Part model, mm, in its own coordinate system. Face numbers are marked on the shaded views. A direction names the side the tool comes from. Round coordinates to 2 decimals unless told otherwise and drop trailing zeros. Loops run counter-clockwise (first coordinate to the right, second up) from the corner with the lowest first, then second, coordinate; pieces in that order, holes last. Notation, with made-up numbers: (74, 50) - (99, 50) arc R28 cw to (99, 75) - close; hole circle Ø9 at (20, 45). An arc over 180 degrees is marked (long way). Put each result on its own line as item: value.
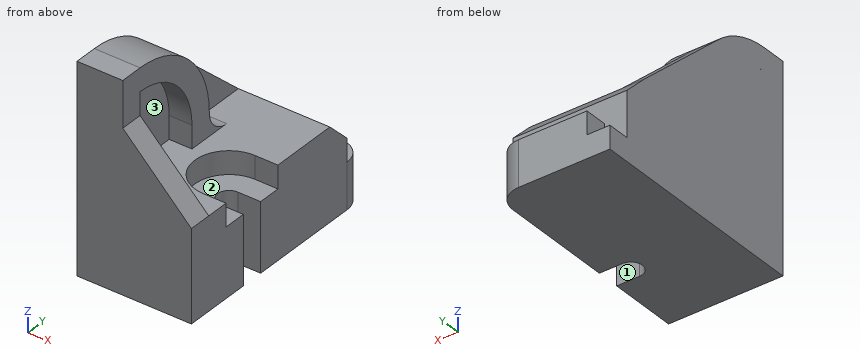
from build123d import *

# Parameters (mm, degrees)
BOSS_EXTRUDE1_DEPTH = 4
CUT_EXTRUDE1_DEPTH  = 1
SKETCH3_W           = 1
SKETCH3_H           = 1
CUT_EXTRUDE2_DEPTH  = 3
SKETCH4_W           = 2
SKETCH4_H           = 1
CUT_EXTRUDE4_DEPTH  = 6
CUT_EXTRUDE5_DEPTH  = 6
BOSS_EXTRUDE2_DEPTH = 1
BOSS_EXTRUDE3_DEPTH = 2
BOSS_EXTRUDE4_DEPTH = 1


with BuildPart() as part:
    # Sketch1 → Boss-Extrude1 (new body)
    with BuildSketch(Plane.XY):
        with BuildLine():
            Line((0, 9), (5, 9))
            ThreePointArc((5, 9), (4.707106781, 9.707106781), (4, 10))
            Line((4, 10), (0, 10))
            Line((0, 10), (0, 9))
        make_face()
        with BuildLine():
            ThreePointArc((4, 4), (3.5, 3.5), (4, 3))
            Line((4, 3), (5, 3))
            Line((5, 3), (5, 0))
            Line((5, 0), (0, 0))
            Line((0, 0), (0, 9))
            Line((0, 9), (5, 9))
            Line((5, 9), (5, 4))
            Line((5, 4), (4, 4))
        make_face()
    extrude(amount=BOSS_EXTRUDE1_DEPTH)

    # Sketch2 → Cut-Extrude1 (cut)
    with BuildSketch(Plane.XY.offset(4)):
        with BuildLine():
            Line((5, 3), (5, 2))
            Line((5, 2), (4, 2))
            ThreePointArc((4, 2), (2.5, 3.5), (4, 5))
            Line((4, 5), (5, 5))
            Line((5, 5), (5, 4))
            Line((5, 4), (4, 4))
            ThreePointArc((4, 4), (3.5, 3.5), (4, 3))
            Line((4, 3), (5, 3))
        make_face()
    extrude(amount=-CUT_EXTRUDE1_DEPTH, mode=Mode.SUBTRACT)

    # Sketch3 → Cut-Extrude2 (cut)
    with BuildSketch(Plane.XY.offset(4)):
        with Locations((0.5, 9.5)):
            Rectangle(SKETCH3_W, SKETCH3_H)
    extrude(amount=-CUT_EXTRUDE2_DEPTH, mode=Mode.SUBTRACT)

    # Sketch4 → Cut-Extrude4 (cut, through all)
    with BuildSketch(Plane.ZY):
        with Locations((3, 9.5)):
            Rectangle(SKETCH4_W, SKETCH4_H)
    extrude(amount=-CUT_EXTRUDE4_DEPTH, mode=Mode.SUBTRACT)

    # Sketch5 → Cut-Extrude5 (cut, through all)
    with BuildSketch(Plane(origin=(5, 0, 0), x_dir=(0, 0, -1), z_dir=(1, 0, 0))):
        Polygon((-3, 9), (-4, 8), (-4, 9), align=None)
    extrude(amount=-CUT_EXTRUDE5_DEPTH, mode=Mode.SUBTRACT)

    # Sketch6 → Boss-Extrude2 (add)
    with BuildSketch(Plane.XZ):
        Polygon((0, 4), (0, 9), (2, 9), (2, 7), (5, 4), align=None)
    extrude(amount=-BOSS_EXTRUDE2_DEPTH)

    # Sketch7 → Boss-Extrude3 (add)
    with BuildSketch(Plane.ZY):
        with BuildLine():
            Line((8, 1), (9, 1))
            ThreePointArc((9, 1), (7.828427125, 3.828427125), (5, 5))
            ThreePointArc((5, 5), (4.292893219, 5.292893219), (4, 6))
            Line((4, 6), (4, 4))
            Line((4, 4), (5, 4))
            ThreePointArc((5, 4), (7.121320344, 3.121320344), (8, 1))
        make_face()
    extrude(amount=-BOSS_EXTRUDE3_DEPTH)

    # Sketch9 → Boss-Extrude4 (add)
    with BuildSketch(Plane.ZY):
        Polygon((4, 8), (7.828427125, 3.828427125), (8, 1), (4, 1), align=None)
    extrude(amount=-BOSS_EXTRUDE4_DEPTH)


solid = part.part
1. Probe line 1 along Z through (x, y) = (4.05, 7); line 2 along Z through (x, y) = (1.9, 3.25); line 3 along X through (y, z) = (3.75, 4.75). List the from-to ranges inside material, lowest first. Write a range as [from, to].
A:
line 1: z = [0, 4]
line 2: z = [0, 4], [6.98, 8.31]
line 3: x = [0, 1]
2. Pin check, flat tips, straight feed: P1, Ø0.8, axis at x = 4.5, z = 3.5, coming from the +Y side; P2, Ø0.5, axis at y = 9.5, z = 1.5, coming from the -X side; P3, Ø0.8, axis at x = 4.5, z = 2, coming from the +Y side (3 decimals). Stop position of each tip, or through.
A:
P1: stops at y = 8.9
P2: stops at x = 1
P3: stops at y = 9.995
3. Band-saw the part on C-C (y = 2.5). List the corners of the cut face in (x, z).
A:
outline: (0, 0) - (5, 0) - (5, 3) - (2.88, 3) - (2.88, 4) - (1, 4) - (1, 7.6) - (2, 7.6) - (2, 8.71) - (0, 8.71) - close
4. Band-saw the part on D-D (x = 3.8). List the corners of the cut face in (y, z).
A:
outline: (0, 0) - (3.04, 0) - (3.04, 3) - (2.01, 3) - (2.01, 4) - (1, 4) - (1, 5.2) - (0, 5.2) - close; (3.96, 0) - (10, 0) - (10, 2) - (9, 2) - (9, 3) - (8, 4) - (4.99, 4) - (4.99, 3) - (3.96, 3) - close
5. Tool access for the marked faces 1, 2 and 3: list every direction of +Z, -Z, +X, -X, +Y, -Y with a clear straight run to the whole face (end or side of a thin tool).
A:
face 1: +Z, -Z, +X
face 2: +Z, +X
face 3: +X
6. Band-saw the part on A-A (x = 0.85). List the corners of the cut face in (y, z), plus the area to 3 significant figures.
A:
outline: (0, 0) - (10, 0) - (10, 1) - (9, 1) - (9, 3) - (8, 4) - (3.83, 7.83) arc R4 ccw to (1, 9) - (0, 9) - close; hole (1, 8) - (1.36, 7.98) arc R3 ccw to start
area: 62.6 mm²
7. Band-saw the part on B-B (z = 3.25). List the corners of the cut face in (x, y).
A:
outline: (0, 0) - (5, 0) - (5, 2) - (4, 2) arc R1.5 cw to (4, 5) - (5, 5) - (5, 8.75) - (0, 8.75) - close
